Part print with two shaded views. Sizes in mm from the minimum x, y, z corner. Round coordinates to 2 decimals unless told otherwise and drop trailing zeros. Order: outer loops, then holes, each group sorted by start corner. A loop starts at its lowest first (then second) coordinate and runs counter-clockwise, first axis right, second up. Notation, with made-up numbers: (-15.75, 66) -> (8.25, 66) arc R18 ccw to (8.25, 92) -> close; hole circle Ø4 at (65.25, 49.25). An arc over 180 degrees is marked (long way). Answer as a JSON object with one key per item and string values.
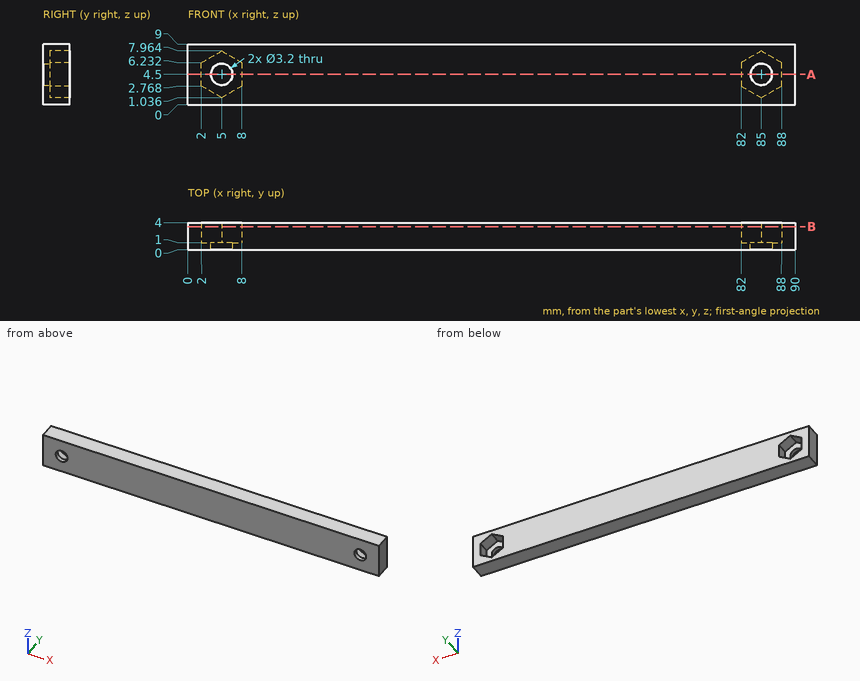
1) Cut at A-A, the plane z = 4.5. Give the cut face in (x, y).
Checked values:
{"outline": "(0, 0) -> (3.4, 0) -> (3.4, 1) -> (2, 1) -> (2, 4) -> (0, 4) -> close; (6.6, 0) -> (83.4, 0) -> (83.4, 1) -> (82, 1) -> (82, 4) -> (8, 4) -> (8, 1) -> (6.6, 1) -> close; (86.6, 0) -> (90, 0) -> (90, 4) -> (88, 4) -> (88, 1) -> (86.6, 1) -> close"}
2) Flat gauge pin, fed straight in: pin 1 Ø4 at (x, z) = (5, 4.5) entering from +Y. Where does the tip first touch, or does it go through?
Checked values:
{"pin 1": "stops at y = 1"}
3) Cut at B-B, the plane y = 3.4. Give the cut face in (x, z).
Checked values:
{"outline": "(0, 0) -> (90, 0) -> (90, 9) -> (0, 9) -> close; hole (2, 2.77) -> (5, 1.04) -> (8, 2.77) -> (8, 6.23) -> (5, 7.96) -> (2, 6.23) -> close; hole (82, 2.77) -> (85, 1.04) -> (88, 2.77) -> (88, 6.23) -> (85, 7.96) -> (82, 6.23) -> close"}
4) Probe L1, parallel to X at y = 0.85, z = 4.5; L2, parallel to X at y = 2.05, z = 5.75; L3, parallel to Z at x = 85, y = 2.85. List the from-to ranges inside material, lowest first. Write a range as from..to.
Checked values:
{"L1": "x = 0..3.4, 6.6..83.4, 86.6..90", "L2": "x = 0..2, 8..82, 88..90", "L3": "z = 0..1.04, 7.96..9"}
